Verification items for the finished model (mm, model axes). Face numbers are marked on the shaded views. A direction names the side the tool comes from. Round coordinates to 2 decimals unless told otherwise and drop trailing zeros. Write each loop counter-clockwise with the first axis right and the second up, starting at its lowest first coordinate (ties: lowest second). Pieces come first, ordered by that corner, then holes.
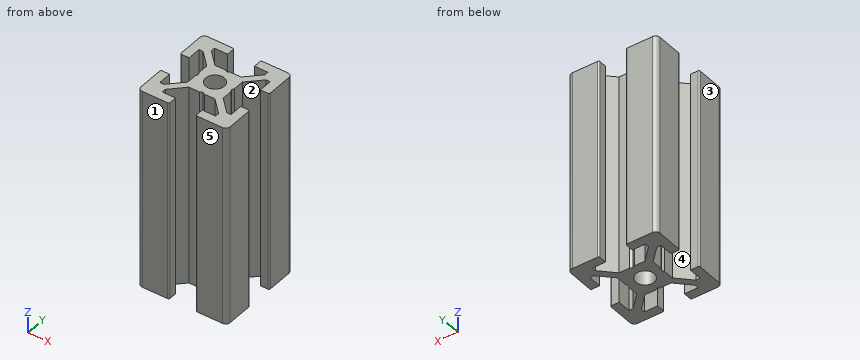
from build123d import *

# Parameters (mm, degrees)
BOSS_EXTRUDE1_DEPTH = 45
SKETCH2_W           = 400
SKETCH2_H           = 2.1


with BuildPart() as part:
    # Sketch1 → Boss-Extrude1 (new body)
    with BuildSketch(Plane.XY):
        with BuildLine():
            Line((-10, 9), (-10, 3.29999995))
            ThreePointArc((-10, 3.29999995), (-9.912132049, 3.087867916), (-9.7, 3))
            Line((-9.7, 3), (-8, 3))
            Line((-8, 3), (-8, 6))
            Line((-8, 6), (-7.060677, 6))
            Line((-7.060677, 6), (-4, 2.93932965))
            Line((-4, 2.93932965), (-4, 0.519615242))
            Line((-4, 0.519615242), (-3.699996283, -6.437e-06))
            Line((-3.699996283, -6.437e-06), (-4, -0.519628117))
            Line((-4, -0.519628117), (-4, -2.93933725))
            Line((-4, -2.93933725), (-7.0606695, -6))
            Line((-7.0606695, -6), (-8, -6))
            Line((-8, -6), (-8, -3))
            Line((-8, -3), (-9.7, -3))
            ThreePointArc((-9.7, -3), (-9.912132049, -3.087867916), (-10, -3.29999995))
            Line((-10, -3.29999995), (-10, -9))
            ThreePointArc((-10, -9), (-9.707106781, -9.707106781), (-9, -10))
            Line((-9, -10), (-3.29999995, -10))
            ThreePointArc((-3.29999995, -10), (-3.087867916, -9.912132049), (-3, -9.7))
            Line((-3, -9.7), (-3, -8))
            Line((-3, -8), (-6, -8))
            Line((-6, -8), (-6, -7.0606515))
            Line((-6, -7.0606515), (-2.9393489, -4))
            Line((-2.9393489, -4), (-0.519615242, -4))
            Line((-0.519615242, -4), (6.437e-06, -3.699996283))
            Line((6.437e-06, -3.699996283), (0.519628117, -4))
            Line((0.519628117, -4), (2.9393227, -4))
            Line((2.9393227, -4), (6, -7.060677))
            Line((6, -7.060677), (6, -8))
            Line((6, -8), (3, -8))
            Line((3, -8), (3, -9.7))
            ThreePointArc((3, -9.7), (3.087867916, -9.912132049), (3.29999995, -10))
            Line((3.29999995, -10), (9, -10))
            ThreePointArc((9, -10), (9.707106781, -9.707106781), (10, -9))
            Line((10, -9), (10, -3.29999995))
            ThreePointArc((10, -3.29999995), (9.912132049, -3.087867916), (9.7, -3))
            Line((9.7, -3), (8, -3))
            Line((8, -3), (8, -6))
            Line((8, -6), (7.0606435, -6))
            Line((7.0606435, -6), (4, -2.9393482))
            Line((4, -2.9393482), (4, -0.519615242))
            Line((4, -0.519615242), (3.699996283, 6.437e-06))
            Line((3.699996283, 6.437e-06), (4, 0.519628117))
            Line((4, 0.519628117), (4, 2.9393401))
            Line((4, 2.9393401), (7.060651, 6))
            Line((7.060651, 6), (8, 6))
            Line((8, 6), (8, 3))
            Line((8, 3), (9.7, 3))
            ThreePointArc((9.7, 3), (9.912132049, 3.087867916), (10, 3.29999995))
            Line((10, 3.29999995), (10, 9))
            ThreePointArc((10, 9), (9.707106781, 9.707106781), (9, 10))
            Line((9, 10), (3.29999995, 10))
            ThreePointArc((3.29999995, 10), (3.087867916, 9.912132049), (3, 9.7))
            Line((3, 9.7), (3, 8))
            Line((3, 8), (6, 8))
            Line((6, 8), (6, 7.060669))
            Line((6, 7.060669), (2.9393308, 4))
            Line((2.9393308, 4), (0.519615242, 4))
            Line((0.519615242, 4), (-6.437e-06, 3.699996283))
            Line((-6.437e-06, 3.699996283), (-0.519628117, 4))
            Line((-0.519628117, 4), (-2.93935655, 4))
            Line((-2.93935655, 4), (-6, 7.0606435))
            Line((-6, 7.0606435), (-6, 8))
            Line((-6, 8), (-3, 8))
            Line((-3, 8), (-3, 9.7))
            ThreePointArc((-3, 9.7), (-3.087867966, 9.912132034), (-3.3, 10))
            Line((-3.3, 10), (-9, 10))
            ThreePointArc((-9, 10), (-9.707106781, 9.707106781), (-10, 9))
        make_face()
    extrude(amount=-BOSS_EXTRUDE1_DEPTH)

    # Sketch2 → Cut-Revolve1 (revolve, cut)
    with BuildSketch(Plane(origin=(0, 0, 0), x_dir=(0, 0, -1), z_dir=(1, 0, 0)), mode=Mode.PRIVATE) as cut_revolve1_sk:
        with Locations((200, 1.05)):
            Rectangle(SKETCH2_W, SKETCH2_H)
    revolve(cut_revolve1_sk.sketch.rotate(Axis((0, 0, -400), (0, 0, 1)), 270), axis=Axis((0, 0, -400), (0, 0, 1)), mode=Mode.SUBTRACT)


solid = part.part
Q1. Tool access check on the marked faces 4 and 5. Record the directions out of +Z, -Z, +X, -X, +Y, -Y that give a thin tool (end or side, any length) a straight path to the whole face; none if there is none.
Recorded:
face 4: +Z, -Z
face 5: +Z, -Z, +X, -X, -Y
Q2. Depth check by flat-ended pin: P1, Ø0.7, axis at x = 2, z = -27.5, coming from the +Y side; P2, Ø2, axis at y = -1.5, z = -5.5, coming from the +X side; P3, Ø1.9, axis at y = -1.5, z = -31, coming from the -X side. Enter the tip coordinate at first touch or a pass-through.
Recorded:
P1: stops at y = 4
P2: stops at x = 4
P3: stops at x = -4
Q3. Sectioned sample at D-D (x = 1.5). Enter the section's corners in (y, z).
Recorded:
outline: (-4, -45) - (-1.47, -45) - (-1.47, 0) - (-4, 0) - close; (1.47, -45) - (4, -45) - (4, 0) - (1.47, 0) - close
Q4. Release check for a two-part mould opening along Y. For the marked faces 1, 2 and 3 record: released by +Y, released by -Y, zero draft, split by the parting line, or undercut.
Recorded:
face 1: released by -Y
face 2: undercut
face 3: zero draft
Q5. Material ranges on line 1 along X through (y, z) = (0, -11.5); line 2 along X through (y, z) = (-5.5, -41), recorded low to high.
Recorded:
line 1: x = -3.7 to -2.1, 2.1 to 3.7
line 2: x = -10 to -8, -6.56 to -4.44, 4.44 to 6.56, 8 to 10
Q6. Sectioned sample at A-A (y = 8.5). Enter the section's corners in (x, z), plus the area to 3 significant figures.
Recorded:
outline: (-10, -45) - (-3, -45) - (-3, 0) - (-10, 0) - close; (3, -45) - (10, -45) - (10, 0) - (3, 0) - close
area: 630 mm2
Q7. Sectioned sample at B-B (x = 4.75). Enter the section's corners in (y, z), plus the area to 3 significant figures.
Recorded:
outline: (-10, -45) - (-8, -45) - (-8, 0) - (-10, 0) - close; (-5.81, -45) - (-3.69, -45) - (-3.69, 0) - (-5.81, 0) - close; (3.69, -45) - (5.81, -45) - (5.81, 0) - (3.69, 0) - close; (8, -45) - (10, -45) - (10, 0) - (8, 0) - close
area: 371 mm2
